Read the model definition and answer for the solid it produces. Units are mm, in the model's axes. A direction names the side the tool comes from. Coordinates: 2 decimals unless noted, no trailing zeros. Order: outer loops, then holes, each group sorted by start corner. A loop starts at its lowest first (then second) coordinate and runs counter-clockwise, first axis right, second up. Notation, with made-up numbers: (85, 85.25) -> (115, 85.25) arc R20 ccw to (115, 104.25) -> close; hole circle Ø10 at (-4.75, -16.75). An arc over 180 degrees is marked (long way). Answer as a JSON object with one key per item and string values. Group by question number.
1) Determine the mould class of faces 1 (the flat face through (17, 13, -0.81)), 2 (the flat face through (23.6, 0, -0.5)), 3 (the cylindrical face through (36.136, 13.991, -12.556)), 4 (the cylindrical face through (36.08, 12.68, -0.44)) for opening direction Z: released by +Z, released by -Z, zero draft, split by the parting line, or undercut.
2) Consider L1, parallel to Y at x = 15, z = -0.5; L2, parallel to Z at x = 24.5, y = 13; L3, parallel to X at y = 8.75, z = -18. Determine where each line is inside the solid, lowest interval first.
3) Section C-C on y = 12.5 is taken. Determine the outline of the cut face in (x, z), and give its area (3 significant figures).
4) A tool of negligible diameter and unlimited length cuts with its end or side. For faces 5 (the flat face through (35.737, 13, -9)), 6 (the flat face through (36, 13, -20.5)), from which of +Z, -Z, +X, -X, +Y, -Y can it reach the whole face along a straight path? Write none if from no direction.
5) Section A-A on y = 7 is taken. Determine the outline of the cut face in (x, z), and give its area (3 significant figures).
6) Section B-B on x = 15 is taken. Determine the outline of the cut face in (y, z), and give its area (3 significant figures).
7) Section D-D on z = -14.5 is taken. Determine the outline of the cut face in (x, y).
8) Given pin 1 (5.5 mm diameter, centred on y = 13, z = -13.5, fed in from -X); pin 2 (5.5 mm diameter, centred on y = 12.5, z = -14.5, fed in from +X); pin 3 (3 mm diameter, centred on x = 25, y = 7, fed in from -Z); pin 4 (5 mm diameter, centred on x = 18.5, y = 14.5, fed in from -Z), each flat-ended and moving along its own axis, determine where each tip first touches the part or whether it passes through.
from build123d import *

# Parameters (mm, degrees)
SKETCH1_W          = 35
SKETCH1_H          = 25
BASE_FLANGE1_DEPTH = 0.81
EDGE_FLANGE1_DEPTH = 25
CUT_EXTRUDE1_REACH = 57.943
SKETCH9_R          = 2
CUT_EXTRUDE2_REACH = 57.921
SKETCH11_R         = 2.45


# Sheet-metal steps are written as plain solids
with BuildPart() as part:
    # Sketch1 → Base-Flange1 (new body)
    with BuildSketch(Plane.XY):
        with Locations((17.5, 12.5)):
            Rectangle(SKETCH1_W, SKETCH1_H)
    extrude(amount=-BASE_FLANGE1_DEPTH)

    # Edge-Flange1 section (across the edge) → Edge-Flange1 (add)
    with BuildSketch(Plane(origin=(35.7366, 25, -0.81), x_dir=(-1, 0, 0), z_dir=(0, -1, 0))):
        with BuildLine():
            Line((-0.81, 0.7366), (-0.81, 34.19))
            Line((-0.81, 34.19), (0, 34.19))
            Line((0, 34.19), (0, 0.7366))
            ThreePointArc((0, 0.7366), (0.215745145, 0.215745145), (0.7366, 0))
            Line((0.7366, 0), (0.7366, -0.81))
            ThreePointArc((0.7366, -0.81), (-0.357011348, -0.357011348), (-0.81, 0.7366))
        make_face()
    extrude(amount=EDGE_FLANGE1_DEPTH)

    # Sketch9 → Cut-Extrude1 (cut, up to next)
    with BuildSketch(Plane(origin=(0, 0, -0.81), x_dir=(-1, 0, 0), z_dir=(0, 0, -1)), mode=Mode.PRIVATE) as cut_extrude1_sk1:
        with Locations((-25, 18)):
            Circle(SKETCH9_R)
    cut_extrude1_tool1 = extrude(cut_extrude1_sk1.sketch, amount=-CUT_EXTRUDE1_REACH, mode=Mode.PRIVATE) & part.part
    # Sketch9 → Cut-Extrude1 (cut, up to next)
    with BuildSketch(Plane(origin=(0, 0, -0.81), x_dir=(-1, 0, 0), z_dir=(0, 0, -1)), mode=Mode.PRIVATE) as cut_extrude1_sk2:
        with Locations((-25, 7)):
            Circle(SKETCH9_R)
    cut_extrude1_tool2 = extrude(cut_extrude1_sk2.sketch, amount=-CUT_EXTRUDE1_REACH, mode=Mode.PRIVATE) & part.part
    # Sketch9 → Cut-Extrude1 (cut, up to next)
    with BuildSketch(Plane(origin=(0, 0, -0.81), x_dir=(-1, 0, 0), z_dir=(0, 0, -1)), mode=Mode.PRIVATE) as cut_extrude1_sk3:
        with Locations((-15, 18)):
            Circle(SKETCH9_R)
    cut_extrude1_tool3 = extrude(cut_extrude1_sk3.sketch, amount=-CUT_EXTRUDE1_REACH, mode=Mode.PRIVATE) & part.part
    # Sketch9 → Cut-Extrude1 (cut, up to next)
    with BuildSketch(Plane(origin=(0, 0, -0.81), x_dir=(-1, 0, 0), z_dir=(0, 0, -1)), mode=Mode.PRIVATE) as cut_extrude1_sk4:
        with Locations((-15, 7)):
            Circle(SKETCH9_R)
    cut_extrude1_tool4 = extrude(cut_extrude1_sk4.sketch, amount=-CUT_EXTRUDE1_REACH, mode=Mode.PRIVATE) & part.part
    add(cut_extrude1_tool1.solids().sort_by_distance((25, 18, -0.81))[0], mode=Mode.SUBTRACT)
    add(cut_extrude1_tool2.solids().sort_by_distance((25, 7, -0.81))[0], mode=Mode.SUBTRACT)
    add(cut_extrude1_tool3.solids().sort_by_distance((15, 18, -0.81))[0], mode=Mode.SUBTRACT)
    add(cut_extrude1_tool4.solids().sort_by_distance((15, 7, -0.81))[0], mode=Mode.SUBTRACT)

    # Sketch11 → Cut-Extrude2 (cut, up to next)
    with BuildSketch(Plane.ZY.offset(-35.7366), mode=Mode.PRIVATE) as cut_extrude2_sk1:
        with Locations(Location((-14.5, 12.5, 0), (0, 0, 180))):
            Circle(SKETCH11_R)
    cut_extrude2_tool1 = extrude(cut_extrude2_sk1.sketch, amount=-CUT_EXTRUDE2_REACH, mode=Mode.PRIVATE) & part.part
    # Sketch11 → Cut-Extrude2 (cut, up to next)
    with BuildSketch(Plane.ZY.offset(-35.7366), mode=Mode.PRIVATE) as cut_extrude2_sk2:
        Polygon((-9.5, 25), (-20.5, 16.25), (-20.5, 8.75), (-9.5, 0), (-14.5, 0), (-39.5, 0), (-39.5, 25), (-14.5, 25), align=None)
    cut_extrude2_tool2 = extrude(cut_extrude2_sk2.sketch, amount=-CUT_EXTRUDE2_REACH, mode=Mode.PRIVATE) & part.part
    add(cut_extrude2_tool1.solids().sort_by_distance((35.7366, 12.5, -14.5))[0], mode=Mode.SUBTRACT)
    add(cut_extrude2_tool2.solids().sort_by_distance((35.7366, 12.5, -27.781546))[0], mode=Mode.SUBTRACT)


solid = part.part
Worked answers:
{
 "1": {"face 1": "released by -Z", "face 2": "zero draft", "face 3": "undercut", "face 4": "released by +Z"},
 "2": {"L1": "y = 0 to 5, 9 to 16, 20 to 25", "L2": "z = -0.81 to 0", "L3": "x = 35.74 to 36.55"},
 "3": {"outline": "(0, -0.81) -> (35, -0.81) arc R0.74 cw to (35.74, -1.55) -> (35.74, -12.05) -> (36.55, -12.05) -> (36.55, -1.55) arc R1.55 ccw to (35, 0) -> (0, 0) -> close; (35.74, -20.5) -> (36.55, -20.5) -> (36.55, -16.95) -> (35.74, -16.95) -> close", "area": "41.2 mm²"},
 "4": {"face 5": "-Z, -X, +Y, -Y", "face 6": "-Z, +X, -X, +Y, -Y"},
 "5": {"outline": "(0, -0.81) -> (13, -0.81) -> (13, 0) -> (0, 0) -> close; (17, -0.81) -> (23, -0.81) -> (23, 0) -> (17, 0) -> close; (27, -0.81) -> (35, -0.81) arc R0.74 cw to (35.74, -1.55) -> (35.74, -18.3) -> (36.55, -18.3) -> (36.55, -1.55) arc R1.55 ccw to (35, 0) -> (27, 0) -> close", "area": "36.9 mm²"},
 "6": {"outline": "(0, -0.81) -> (5, -0.81) -> (5, 0) -> (0, 0) -> close; (9, -0.81) -> (16, -0.81) -> (16, 0) -> (9, 0) -> close; (20, -0.81) -> (25, -0.81) -> (25, 0) -> (20, 0) -> close", "area": "13.8 mm²"},
 "7": {"outline": "(35.74, 3.98) -> (36.55, 3.98) -> (36.55, 10.05) -> (35.74, 10.05) -> close; (35.74, 14.95) -> (36.55, 14.95) -> (36.55, 21.02) -> (35.74, 21.02) -> close"},
 "8": {"pin 1": "stops at x = 35.74", "pin 2": "stops at x = 36.55", "pin 3": "passes through", "pin 4": "stops at z = -0.81"}
}
